For this review, take the finished solid that the model builds, in its own axes (mm). A direction names the side the tool comes from. Coordinates: 2 decimals unless noted, no trailing zeros. Order: outer loops, then holes, each group sorted by start corner. A loop starts at its lowest first (then second) coordinate and runs counter-clockwise, first axis right, second up. Notation, with made-up numbers: (67.25, -26) -> (88.25, -26) arc R17 ccw to (88.25, 2) -> close; hole circle Ø7 at (-14, 32). An arc over 180 degrees is marked (long way). Return JSON: item names as keys, results as strings. Group by question number.
Item 1: Take a section at C-C (x = -51.5). Write out the cut boundary in (y, z) (3 decimals), then the cut area to 3 significant figures.
Item 2: For line 1 along Z through (x, y) = (-61, 0) (3 decimals); line 2 along X through (y, z) = (-4.5, -0.5) (3 decimals); line 3 along Z through (x, y) = (-33, -1.5), list the stretches that pass through material, from the lowest coordinate up.
Item 3: Insertion check: pin 1 (2 mm diameter, centred on y = -2, z = -3.5, fed in from -X); pin 2 (4 mm diameter, centred on y = 4, z = 2, fed in from -X); pin 3 (2 mm diameter, centred on y = 0.5, z = 4.5, fed in from -X) (3 decimals). Each pin has a flat end and moves straight along its axis. Give the tip position at first contact, or say it passes through.
Item 4: Machinability: for faces 1 (the cylindrical face through (-39.72, -0.69, -3.1)), 2 (the flat face through (-6.35, 0, 4)), 3 (the cylindrical face through (-7.956, -4.394, -3.369)), which of the approach directions +Z, -Z, +X, -X, +Y, -Y give a long, thin tool a straight path to every point of the face, cutting with its end or side? Answer none if there is none.
```python
from build123d import *

# Parameters (mm, degrees)
F2_SIZE = 0.762
F3_R    = 0.254


with BuildPart() as f1:
    # F0 (on Top) → F1 (revolve)
    with BuildSketch(Plane.XY):
        Polygon((-69.85, 0), (0, 0), (0, 3.048), (-6.35, 3.556), (-6.35, 5.5372), (-9.525, 5.5372), (-9.525, 3.175), (-69.85, 3.175), align=None)
    revolve(axis=Axis((-34.925, 0, 0), (1, 0, 0)))

    # F2
    f2_edges = [f1.edges().sort_by_distance(p)[0] for p in [
        (-69.85, -3.175, 0),
    ]]
    chamfer(f2_edges, length=F2_SIZE)

    # F3
    f3_edges = [f1.edges().sort_by_distance(p)[0] for p in [
        (-9.525, -5.5372, 0),
        (-6.35, -5.5372, 0),
        (0, -3.048, 0),
    ]]
    fillet(f3_edges, radius=F3_R)


solid = f1.part
```
Findings below:
{
 "1": {"outline": "circle Ø6.35 at (0, 0)", "area": "31.7 mm2"},
 "2": {"line 1": "z = -3.175 to 3.175", "line 2": "x = -9.525 to -6.35", "line 3": "z = -2.8 to 2.8"},
 "3": {"pin 1": "stops at x = -69.23", "pin 2": "stops at x = -69.79", "pin 3": "stops at x = -9.525"},
 "4": {"face 1": "-X", "face 2": "+X", "face 3": "+X, -X"}
}
